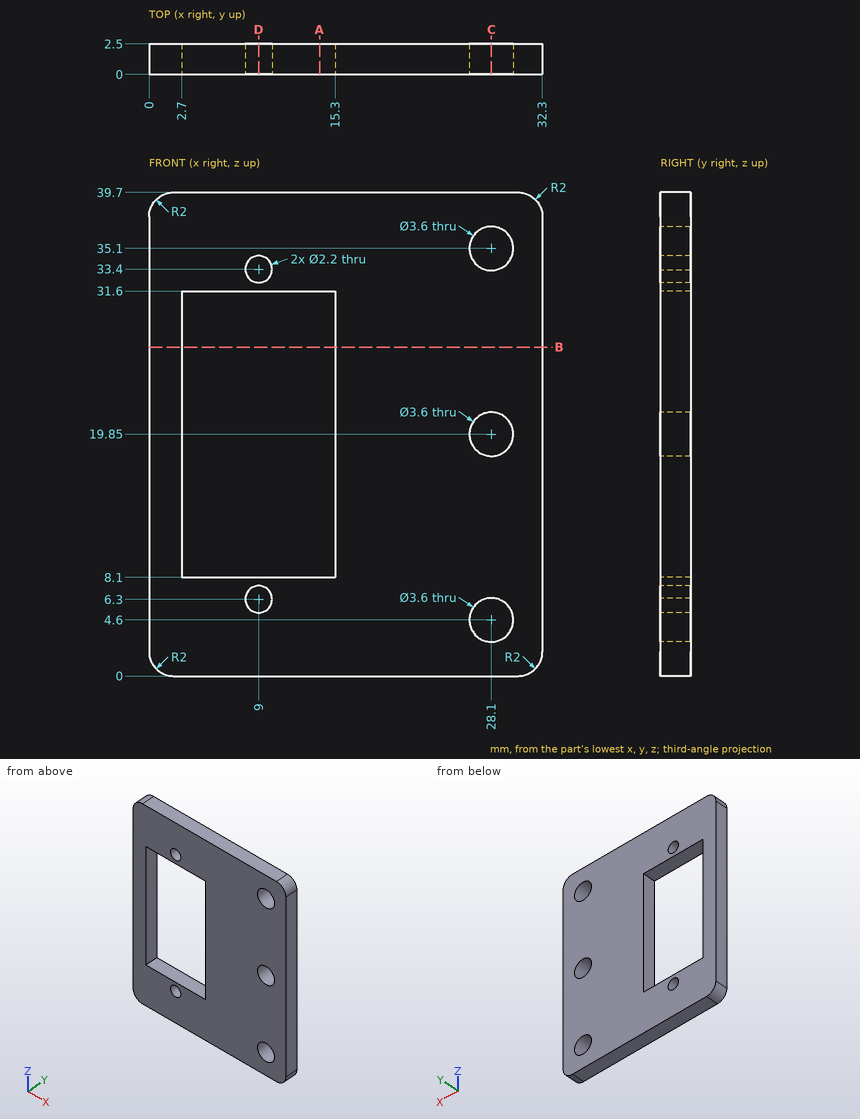
Check sheet for the drawn part. Datum: minimum x, y, z corner. Units: mm. Round coordinates to 2 decimals unless told otherwise and drop trailing zeros. Write each loop counter-clockwise with the first axis right and the second up, starting at its lowest first coordinate (ties: lowest second). Pieces come first, ordered by that corner, then holes. Notation, with made-up numbers: (25.5, 60.5) -> (76.5, 60.5) arc R11 cw to (76.5, 65.5) -> close; hole circle Ø2 at (46, 59). An arc over 180 degrees is marked (long way). Put each result on its own line as item: value.
(1) Sectioned sample at D-D (x = 9). Enter the section's corners in (y, z).
Values found:
outline: (0, 0) -> (2.5, 0) -> (2.5, 5.2) -> (0, 5.2) -> close; (0, 7.4) -> (2.5, 7.4) -> (2.5, 8.1) -> (0, 8.1) -> close; (0, 31.6) -> (2.5, 31.6) -> (2.5, 32.3) -> (0, 32.3) -> close; (0, 34.5) -> (2.5, 34.5) -> (2.5, 39.7) -> (0, 39.7) -> close
(2) Sectioned sample at C-C (x = 28.1). Enter the section's corners in (y, z), plus the area to 4 significant figures.
Values found:
outline: (0, 0) -> (2.5, 0) -> (2.5, 2.8) -> (0, 2.8) -> close; (0, 6.4) -> (2.5, 6.4) -> (2.5, 18.05) -> (0, 18.05) -> close; (0, 21.65) -> (2.5, 21.65) -> (2.5, 33.3) -> (0, 33.3) -> close; (0, 36.9) -> (2.5, 36.9) -> (2.5, 39.7) -> (0, 39.7) -> close
area: 72.25 mm^2
(3) Go/stop test with a flat-tipped pin: pin 1 Ø2 at (x, z) = (28.1, 19.85) entering from +Y. Record where the tip stops, or that it passes through.
Values found:
pin 1: passes through
(4) Sectioned sample at B-B (z = 27). Enter the section's corners in (x, y).
Values found:
outline: (0, 0) -> (2.7, 0) -> (2.7, 2.5) -> (0, 2.5) -> close; (15.3, 0) -> (32.3, 0) -> (32.3, 2.5) -> (15.3, 2.5) -> close
(5) Sectioned sample at A-A (x = 14). Enter the section's corners in (y, z).
Values found:
outline: (0, 0) -> (2.5, 0) -> (2.5, 8.1) -> (0, 8.1) -> close; (0, 31.6) -> (2.5, 31.6) -> (2.5, 39.7) -> (0, 39.7) -> close
(6) Material ranges on line 1 (Z direction, x = 28.1, y = 0.65); line 2 (Z direction, x = 11, y = 0.85); line 3 (X direction, y = 0.55, z = 26.5), recorded low to high.
Values found:
line 1: z = 0 to 2.8, 6.4 to 18.05, 21.65 to 33.3, 36.9 to 39.7
line 2: z = 0 to 8.1, 31.6 to 39.7
line 3: x = 0 to 2.7, 15.3 to 32.3
